Geometry: final body of the model. Coordinates: model frame, mm. A direction names the side the tool comes from. Coordinates: 2 decimals unless noted, no trailing zeros. Write each loop counter-clockwise with the first axis right and the second up, starting at its lowest first coordinate (ties: lowest second). Pieces come first, ordered by that corner, then holes.
from build123d import *

# Parameters (mm, degrees)
PAD001_DEPTH           = 21
LINEARPATTERN002_COUNT = 2
LINEARPATTERN002_PITCH = 42


with BuildPart() as part:
    # Sketch004 → Pad001 (new body)
    with BuildSketch(Plane.XY):
        with BuildLine():
            Line((-38, -20.75), (38, -20.75))
            ThreePointArc((38, -20.75), (40.65165, -19.65165), (41.75, -17))
            Line((41.75, -17), (41.75, 17))
            ThreePointArc((41.75, 17), (40.65165, 19.65165), (38, 20.75))
            Line((38, 20.75), (-38, 20.75))
            ThreePointArc((-38, 20.75), (-40.65165, 19.65165), (-41.75, 17))
            Line((-41.75, 17), (-41.75, -17))
            ThreePointArc((-41.75, -17), (-40.65165, -19.65165), (-38, -20.75))
        make_face()
    extrude(amount=PAD001_DEPTH)

    # SubtractivePipe001: sweep along a path in Sketch004
    with BuildLine(Plane.XY) as subtractivepipe001_path:
        Line((-38, -20.75), (38, -20.75))
        ThreePointArc((38, -20.75), (40.65165, -19.65165), (41.75, -17))
        Line((41.75, -17), (41.75, 17))
        ThreePointArc((41.75, 17), (40.65165, 19.65165), (38, 20.75))
        Line((38, 20.75), (-38, 20.75))
        ThreePointArc((-38, 20.75), (-40.65165, 19.65165), (-41.75, 17))
        Line((-41.75, 17), (-41.75, -17))
        ThreePointArc((-41.75, -17), (-40.65165, -19.65165), (-38, -20.75))
    # Sketch005 → SubtractivePipe001 (sweep, cut)
    with BuildSketch(Plane.XZ):
        Polygon((41.75, 4.75), (39.6, 2.6), (39.6, 0.8), (38.8, 0), (41.75, 0), align=None)
    subtractivepipe001 = sweep(path=subtractivepipe001_path.line, mode=Mode.SUBTRACT)

    # LinearPattern002: SubtractivePipe001 ×2
    with Locations(*[(i * LINEARPATTERN002_PITCH, 0, 0) for i in range(1, LINEARPATTERN002_COUNT)]):
        add(subtractivepipe001, mode=Mode.SUBTRACT)


solid = part.part
Item 1: Set-up query: faces 5 (the flat face through (39.6, 0, 2)), 6 (the cylindrical face through (2.88, 18.14, 1.69)), 7 (the flat face through (2.4, 0, 2)), 8 (the flat face through (21, -18.6, 2)). Return all of +Z, -Z, +X, -X, +Y, -Y with unobstructed straight access to the full face (end or side cutting, diameter ignored); none if empty.
Derived:
face 5: -Z, +X, +Y, -Y
face 6: -Z, +Y
face 7: -Z, +Y, -Y
face 8: -Z, +X, -X, -Y
Item 2: Material intervals for probe 1 along Y at (x, z) = (10, 1.75); probe 2 along X at (y, z) = (-8, 3.25); probe 3 along X at (y, z) = (17.5, 7.5), sorted ascending.
Derived:
probe 1: y = -18.6 to 18.6
probe 2: x = -40.25 to 0.25, 1.75 to 40.25
probe 3: x = -41.72 to 41.72
Item 3: Section A-A, the plane x = -30. Output: boundary loops of the cut face in (y, z), plus the area to 3 significant figures.
Derived:
outline: (-20.75, 4.75) - (-18.6, 2.6) - (-18.6, 0.8) - (-17.8, 0) - (17.8, 0) - (18.6, 0.8) - (18.6, 2.6) - (20.75, 4.75) - (20.75, 21) - (-20.75, 21) - close
area: 855 mm2
Item 4: Pull-direction query (X, two-part tool) for faces 1 (the flat face through (41.75, 0, 13)), 2 (the conical face through (-39.73, -18.69, 3.42)), 3 (the flat face through (21, 20, 4)), 4 (the cylindrical face through (2.86, -18.12, 1.69)); classes: released by +X, released by -X, zero draft, split by the parting line, or undercut.
Derived:
face 1: released by +X
face 2: released by -X
face 3: zero draft
face 4: undercut
Item 5: Pin query (flat end, axial travel): pin 1 (0.9 mm diameter, centred on y = 2.5, z = 1.5, fed in from -X); pin 2 (0.5 mm diameter, centred on x = -15.5, z = 1.5, fed in from -Y); pin 3 (1.4 mm diameter, centred on x = 27.5, z = 1.5, fed in from +Y). Return the tip coordinate at first contact, or that it passes through.
Derived:
pin 1: stops at x = -39.6
pin 2: stops at y = -18.6
pin 3: stops at y = 18.6
